```python
from build123d import *

# Parameters (mm, degrees)
SKETCH_1_R          = 1.6
SKETCH_1_R_2        = 15
EXTRUDE_1_DEPTH     = 3
SKETCH_3_W          = 4
SKETCH_3_H          = 20
CUT_EXTRUDE_2_DEPTH = 10
HOLE_WIZARD_1_D     = 3.5
HOLE_WIZARD_3_D     = 3
HOLE_WIZARD_6_D     = 3.8
HOLE_WIZARD_8_D     = 4
SKETCH_25_W         = 30
SKETCH_25_H         = 20
CUT_EXTRUDE_3_DEPTH = 10
FILLET_1_R          = 3
HOLE_WIZARD_9_D     = 3


with BuildPart() as part:
    # 草图1 → 凸台-拉伸1 (new body)
    with BuildSketch(Plane.XY):
        with BuildLine():
            Line((-34, 0), (-34, 40))
            ThreePointArc((-34, 40), (-33.414213562, 41.414213562), (-32, 42))
            Line((-32, 42), (168, 42))
            ThreePointArc((168, 42), (169.414213562, 41.414213562), (170, 40))
            Line((170, 40), (170, 0))
            ThreePointArc((170, 0), (173.807611845, -9.192388155), (183, -13))
            Line((183, -13), (206, -13))
            ThreePointArc((206, -13), (220, -27), (206, -41))
            Line((206, -41), (158, -41))
            ThreePointArc((158, -41), (141.042357362, -36.137397741), (129.238356686, -23.02739726))
            ThreePointArc((129.238356686, -23.02739726), (114.114480821, -6.230209144), (92.387501191, 0))
            Line((92.387501191, 0), (-34, 0))
        make_face()
        with Locations((15.5, 5.5)):
            Circle(SKETCH_1_R, mode=Mode.SUBTRACT)
        with Locations((-15.5, 5.5)):
            Circle(SKETCH_1_R, mode=Mode.SUBTRACT)
        with Locations((-15.5, 36.5)):
            Circle(SKETCH_1_R, mode=Mode.SUBTRACT)
        with Locations((15.5, 36.5)):
            Circle(SKETCH_1_R, mode=Mode.SUBTRACT)
        with Locations((166, 34)):
            Circle(SKETCH_1_R, mode=Mode.SUBTRACT)
        with Locations((166, 10)):
            Circle(SKETCH_1_R, mode=Mode.SUBTRACT)
        with Locations((-30, 10)):
            Circle(SKETCH_1_R, mode=Mode.SUBTRACT)
        with Locations((-30, 34)):
            Circle(SKETCH_1_R, mode=Mode.SUBTRACT)
        with Locations((0, 21)):
            Circle(SKETCH_1_R_2, mode=Mode.SUBTRACT)
        with Locations((166, -37)):
            Circle(SKETCH_1_R, mode=Mode.SUBTRACT)
        with Locations((198, -37)):
            Circle(SKETCH_1_R, mode=Mode.SUBTRACT)
        with Locations((110, 34)):
            Circle(SKETCH_1_R, mode=Mode.SUBTRACT)
        with Locations((110, 10)):
            Circle(SKETCH_1_R, mode=Mode.SUBTRACT)
    extrude(amount=EXTRUDE_1_DEPTH)

    # 草图3 → 切除-拉伸2 (cut)
    with BuildSketch(Plane.XY.offset(3)):
        with Locations((130.178561527, -31)):
            Rectangle(SKETCH_3_W, SKETCH_3_H)
    extrude(amount=-CUT_EXTRUDE_2_DEPTH, mode=Mode.SUBTRACT)

    # 孔1 (through all)
    with Locations(Plane(origin=(0, 0, 0), x_dir=(-1, 0, 0), z_dir=(0, 0, -1))):
        with Locations((-137.178561527, -26)):
            Hole(HOLE_WIZARD_1_D / 2)

    # 孔3 (through all)
    with Locations(Plane(origin=(0, 0, 0), x_dir=(-1, 0, 0), z_dir=(0, 0, -1))):
        with Locations((-164.5, 38.5), (-115.5, 38.5), (-164.5, -19.5)):
            Hole(HOLE_WIZARD_3_D / 2)

    # 孔6 (through all)
    with Locations(Plane(origin=(0, 0, 0), x_dir=(-1, 0, 0), z_dir=(0, 0, -1))):
        with Locations((-166, 24), (-82, 24)):
            Hole(HOLE_WIZARD_6_D / 2)

    # 孔8 (through all)
    with Locations(Plane(origin=(0, 0, 0), x_dir=(-1, 0, 0), z_dir=(0, 0, -1))):
        with Locations((-144.906, -15.042)):
            Hole(HOLE_WIZARD_8_D / 2)

    # 草图25 → 切除-拉伸3 (cut)
    with BuildSketch(Plane(origin=(0, 0, 0), x_dir=(-1, 0, 0), z_dir=(0, 0, -1))):
        with Locations((-46, 22)):
            Rectangle(SKETCH_25_W, SKETCH_25_H)
    extrude(amount=-CUT_EXTRUDE_3_DEPTH, mode=Mode.SUBTRACT)

    # 圆角1
    fillet_1_edges = [part.edges().sort_by_distance(p)[0] for p in [
        (61, 12, 1.5),
        (61, 32, 1.5),
        (31, 32, 1.5),
        (31, 12, 1.5),
    ]]
    fillet(fillet_1_edges, radius=FILLET_1_R)

    # 孔9 (through all)
    with Locations(Plane(origin=(0, 0, 0), x_dir=(-1, 0, 0), z_dir=(0, 0, -1))):
        with Locations((-132.178561527, -22.5)):
            Hole(HOLE_WIZARD_9_D / 2)


solid = part.part
```
Input: part model. Units: mm. Frame: model coordinates. Round coordinates to 2 decimals unless told otherwise and drop trailing zeros. Loops run counter-clockwise (first coordinate to the right, second up) from the corner with the lowest first, then second, coordinate; pieces in that order, holes last. Notation, with made-up numbers: (50.25, 86) - (73.25, 86) arc R20 cw to (73.25, 96) - close; hole circle Ø2 at (45.25, 57.25). An arc over 180 degrees is marked (long way). One line per item, written item: value. Start each with the question number.
(1) Contact query for flat-ended pins moving along their axis: P1, Ø3, axis at x = 137.18, y = -26, coming from the +Z side; P2, Ø4, axis at x = 115.5, y = 38.5, coming from the +Z side. Output: stop coordinate, or through.
(2) Section D-D, the plane z = 1. Count the separate pieces of the cut face and the enclosed holes in it, plus the area to 3 significant figures.
(3) Section A-A, the plane x = -10. Return loops of the section in (y, z), plus the area to 3 significant figures.
(4) Section C-C, the plane y = -9. Return loops of the section in (x, z), plus the area to 3 significant figures.
(5) Ray query, line 1 (Y direction, x = -30, z = 1.25); line 2 (Y direction, x = -15.5, z = 1.1); line 3 (Y direction, x = 35, z = 2.7). Return the intervals inside material, ascending. Write a range as [from, to].
(6) Draft query along X for faces 1 (the cylindrical face through (-3.252, 6.357, 1.479)), 2 (the cylindrical face through (143.71, -37.63, 1.48)), 3 (the flat face through (95, 10, 3)), 4 (the cylindrical face through (173.707, -9.091, 1.479)). Return one class per face: +X half, -X half, draft (parallel to the pull), parting line (faces both ways), or undercut.
(7) Section B-B, the plane x = 65.5. Return loops of the section in (y, z), plus the area to 3 significant figures.
Results below:
1. P1: through
1. P2: z = 3
2. separate pieces: 1
2. enclosed holes: 21
2. area: 10,200 mm^2
3. outline: (0, 0) - (9.82, 0) - (9.82, 3) - (0, 3) - close; (32.18, 0) - (42, 0) - (42, 3) - (32.18, 3) - close
3. area: 58.9 mm^2
4. outline: (118.02, 0) - (173.62, 0) - (173.62, 3) - (118.02, 3) - close
4. area: 167 mm^2
5. line 1: [0, 8.4], [11.6, 32.4], [35.6, 42]
5. line 2: [0, 3.9], [7.1, 34.9], [38.1, 42]
5. line 3: [0, 12], [32, 42]
6. face 1: undercut
6. face 2: -X half
6. face 3: draft
6. face 4: +X half
7. outline: (0, 0) - (42, 0) - (42, 3) - (0, 3) - close
7. area: 126 mm^2
